```python
from build123d import *

# Parameters (mm, degrees)
F1_DEPTH = 15
F0_W     = 120.46892941
F0_H     = 14.3122337759
F2_DEPTH = 65
F3_W     = 50.9056653827
F3_H     = 14.3122337759
F4_DEPTH = 20
F5_R     = 5
F6_ANGLE = 2.4061889728


with BuildPart() as f1:
    # F0 (on Top) → F1 (new body)
    with BuildSketch(Plane.XY):
        Polygon((60.234464705, 45.9222309291), (-60.234464705, 45.9222309291), (-60.234464705, 0), (0, 0), (0, -60.234464705), (60.234464705, -60.234464705), align=None)
    extrude(amount=F1_DEPTH)

    # F0 (on Top) → F2 (join)
    with BuildSketch(Plane.XY):
        with Locations((0, 53.0783478171)):
            Rectangle(F0_W, F0_H)
    extrude(amount=F2_DEPTH)

    # F3 (on face) → F4 (join)
    with BuildSketch(Plane.XY.offset(65)):
        with Locations((-2.0645121112, 53.0783478171)):
            Rectangle(F3_W, F3_H)
    extrude(amount=F4_DEPTH)

    # F5
    f5_edges = [f1.edges().sort_by_distance(p)[0] for p in [
        (0, 45.922231, 15),
        (-60.234465, 45.922231, 40),
        (-43.875905, 45.922231, 65),
        (-27.517345, 45.922231, 75),
        (-2.064512, 45.922231, 85),
        (23.388321, 45.922231, 75),
        (41.811393, 45.922231, 65),
        (60.234465, 45.922231, 40),
        (-60.234465, 22.961115, 15),
        (-30.117232, 0, 15),
        (0, -30.117232, 15),
        (30.117232, -60.234465, 15),
        (60.234465, -7.156117, 15),
    ]]
    fillet(f5_edges, radius=F5_R)


with BuildPart() as f1_1:
    # F6: moved
    add(f1.part.rotate(Axis((60.234464705, 60.234464705, 32.5), (0, 0, -1)), F6_ANGLE))


solid = f1_1.part
```
Input: part model. Units: mm. Frame: model coordinates. A direction names the side the tool comes from. Round coordinates to 2 decimals unless told otherwise and drop trailing zeros. Loops run counter-clockwise (first coordinate to the right, second up) from the corner with the lowest first, then second, coordinate; pieces in that order, holes last. Notation, with made-up numbers: (61.25, 62) -> (79.25, 62) arc R22 ccw to (79.25, 91) -> close; hole circle Ø1 at (28, 49.25). An arc over 180 degrees is marked (long way). Use one line per item in the form item = value. Start each with the question number.
Item 1: Section query A-A on z = 62.5. Return the cut outline in (x, y), then the cut area to 3 significant figures.
Item 2: Section query B-B on y = 58. Return the cut outline in (x, z).
Item 3: Set-up query: faces 4 (the face through (24.665, -58.846, 4.93)), 5 (the face through (23.223, 57.064, 74.86)), 6 (the face through (-27.64, 59.2, 74.86)). Return all of +Z, -Z, +X, -X, +Y, -Y with unobstructed straight access to the full face (end or side cutting, diameter ignored); none if empty.
Item 4: Contact query for flat-ended pins moving along their axis: pin 1 Ø4 at (x, z) = (40, 62) entering from +Y; pin 2 Ø1.5 at (x, y) = (-42.5, 38.5) entering from +Z; pin 3 Ø8.5 at (x, y) = (33, 54) entering from +Z; pin 4 Ø12 at (x, y) = (-29, 17.5) entering from -Z. Output: stop coordinate, or through.
Item 5: Section query C-C on z = 33.5. Return the cut outline in (x, y).
Item 6: Mould query, pull axis Y, two halves, no side actions, for faces 1 (the face through (-60.386, 25.208, 13.496)), 2 (the face through (-1.32, 48.496, 42.913)), 3 (the face through (-0.8, 62.8, 32.5)). Classes: pulls with the +Y half, pulls with the -Y half, needs draft (parallel to the pull), parting line crosses it, or undercut.
Item 7: Material intervals for L1, parallel to Z at x = 30, y = 33; L2, parallel to X at y = 17, z = 6; L3, parallel to Y at x = 8, z = 50, sorted ascending. Write a range as from..to.
Item 8: Section query D-D on z = 77. Return the cut outline in (x, y).
Ans:
q1.outline = (-60.52, 55.99) arc R5 ccw to (-58.2, 51.56) -> (-25.51, 50.18) arc R5 ccw to (-23.05, 49.41) -> (17.82, 47.69) arc R5 ccw to (20.35, 48.26) -> (57.16, 46.71) arc R5 ccw to (59.84, 50.93) -> (60.23, 60.23) -> (-60.13, 65.29) -> close
q1.area = 1,670 mm^2
q2.outline = (-60.43, 0) -> (60.14, 0) -> (60.14, 65) -> (23.26, 65) -> (23.26, 85) -> (-27.69, 85) -> (-27.69, 65) -> (-60.43, 65) -> close
q3.face_4 = +Z, -Z, -X, -Y
q3.face_5 = +Z, +X, -Y
q3.face_6 = +Z, -X, +Y
q4.pin_1 = 61.17
q4.pin_2 = 15
q4.pin_3 = 65
q4.pin_4 = 0
q5.outline = (-60.52, 55.99) arc R5 ccw to (-55.73, 50.78) -> (54.64, 46.14) arc R5 ccw to (59.84, 50.93) -> (60.23, 60.23) -> (-60.13, 65.29) -> close
q6.face_1 = undercut
q6.face_2 = pulls with the -Y half
q6.face_3 = pulls with the +Y half
q7.L1 = 0..15
q7.L2 = -62.16..58.42
q7.L3 = 48.1..62.43
q8.outline = (-27.83, 54.61) arc R5 ccw to (-23.05, 49.41) -> (17.82, 47.69) arc R5 ccw to (23.03, 52.48) -> (23.42, 61.78) -> (-27.44, 63.92) -> close
